Print and shaded views of the part. All mm, measured from the part's lowest x, y and z. Round coordinates to 2 decimals unless told otherwise and drop trailing zeros. Order: outer loops, then holes, each group sorted by start corner. A loop starts at its lowest first (then second) coordinate and runs counter-clockwise, first axis right, second up. Notation, with made-up numbers: (44, 30) -> (89, 30) arc R25 cw to (89, 62) -> close; hole circle Ø8 at (81, 16.5). An arc over 180 degrees is marked (long way). Answer as CSV lines item,"result".
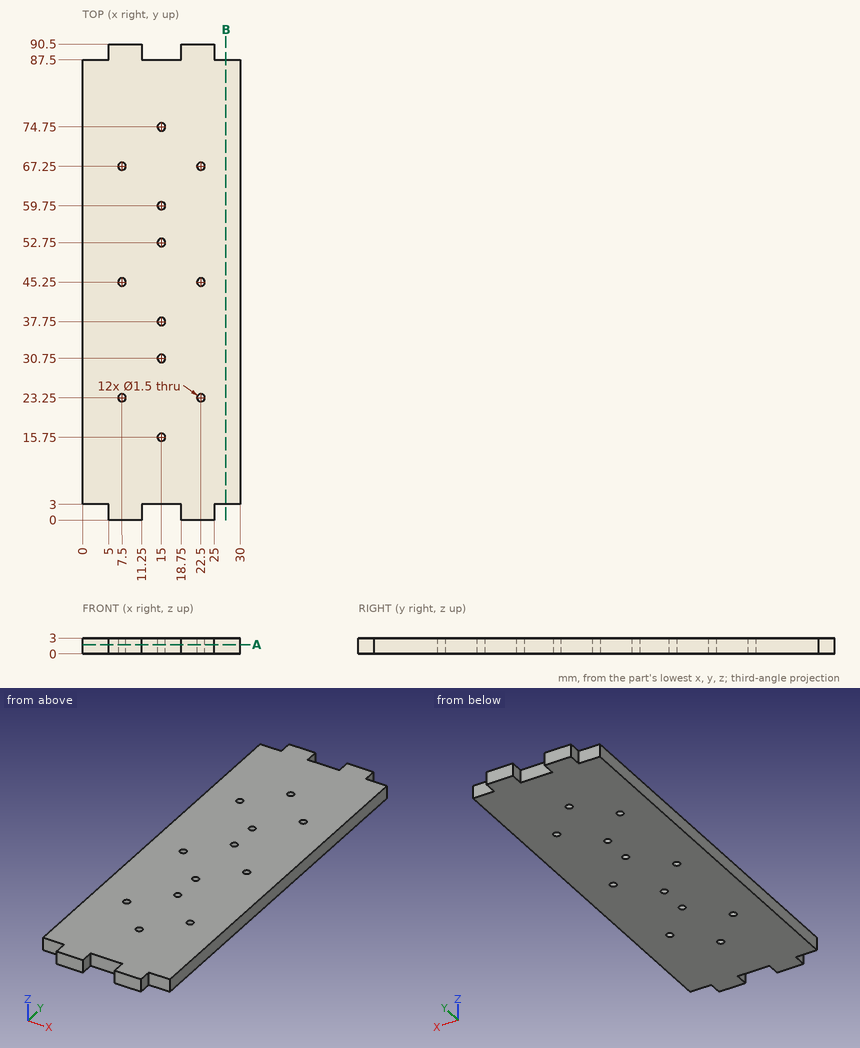
Q1. Saw through at B-B (x = 27.25). Write the cut outline in (y, z), plus the area to 4 significant figures.
Checks:
outline,"(3, 0) -> (87.5, 0) -> (87.5, 3) -> (3, 3) -> close"
area,"253.5 mm²"
Q2. Wall check: L1, parallel to Y at x = 7.5, z = 1.7; L2, parallel to X at y = 45.25, z = 2.05; L3, parallel to X at y = 52.75, z = 1.3. Give the ranges that are in metal, low to high. Write a range as [from, to].
Checks:
L1,"[0, 22.5], [24, 44.5], [46, 66.5], [68, 90.5]"
L2,"[0, 6.75], [8.25, 21.75], [23.25, 30]"
L3,"[0, 14.25], [15.75, 30]"
Q3. Flat gauge pins, fed straight in: pin 1 (1.5 mm diameter, centred on x = 20.5, y = 81, fed in from -Z); pin 2 (1.5 mm diameter, centred on y = 88.5, z = 2, fed in from +X); pin 3 (0.9 mm diameter, centred on x = 27, z = 1, fed in from -Y); pin 4 (0.9 mm diameter, centred on x = 1.5, z = 1, fed in from +Y). Where does each tip first touch, or does it go through?
Checks:
pin 1,"z = 0"
pin 2,"x = 25"
pin 3,"y = 3"
pin 4,"y = 87.5"
Q4. Saw through at A-A (z = 1.75). State how many separate pieces and enclosed holes the cut face has, plus the area to 3 significant figures.
Checks:
separate pieces,"1"
enclosed holes,"12"
area,"2,590 mm²"
